from build123d import *

# Parameters (mm, degrees)
F0_R     = 19.05
F1_DEPTH = 3.302
F2_R     = 8.5345501525
F3_DEPTH = 6.605
F4_R     = 14.0253085835
F4_R_2   = 8.5345501525
F5_DEPTH = 0.762


# Not quite as in the source:
# - a feature names something its author has since deleted; it is built from what else it names


with BuildPart() as f1:
    # F0 (on Front) → F1 (new body, symmetric)
    with BuildSketch(Plane.XZ):
        Circle(F0_R)
    extrude(amount=F1_DEPTH, both=True)

    # F2 (on face) → F3 (cut, through all)
    with BuildSketch(Plane.XZ.offset(3.302)):
        Circle(F2_R)
    extrude(amount=-F3_DEPTH, mode=Mode.SUBTRACT)

    # F4 (on face) → F5 (cut)
    with BuildSketch(Plane.XZ.offset(3.302)):
        Circle(F4_R)
        Circle(F4_R_2, mode=Mode.SUBTRACT)
    extrude(amount=-F5_DEPTH, mode=Mode.SUBTRACT)


solid = f1.part
Verification items for the finished model (mm, model axes). A direction names the side the tool comes from. Coordinates: 2 decimals unless noted, no trailing zeros. Loops run counter-clockwise (first coordinate to the right, second up) from the corner with the lowest first, then second, coordinate; pieces in that order, holes last. Notation, with made-up numbers: (88, 69.25) -> (95, 69.25) arc R22 ccw to (95, 86.25) -> close; hole circle Ø2 at (42, 28.25). An arc over 180 degrees is marked (long way). Answer as a JSON object with one key per item and string values. Group by question number.
Item 1: Scan lines: probe 1 along Z at (x, y) = (0, 0.5); probe 2 along Z at (x, y) = (0, -2.9); probe 3 along Y at (x, z) = (-6.5, 9). Record each from-to range of solid material in increasing order.
Item 2: Sectioned sample at C-C on y = 1.5. Record the boundary of the cut face in (x, z).
Item 3: Tool access check on faces 4 (the cylindrical face through (12.956, -2.926, -5.372)), 5 (the flat face through (-9, -3.302, -11)). Record the directions out of +Z, -Z, +X, -X, +Y, -Y that give a thin tool (end or side, any length) a straight path to the whole face; none if there is none.
Item 4: Mould release check, pull along Z, two halves, no side actions. Record for faces 1 (the cylindrical face through (-15.12, -0.05, -11.59)), 2 (the flat face through (8, 3.302, -4)), 3 (the flat face through (0, -2.54, -9)): +Z half, -Z half, draft (parallel to the pull), parting line (faces both ways), or undercut.
Item 5: Sectioned sample at B-B on z = 0. Record the boundary of the cut face in (x, y).
Item 6: Depth check by flat-ended pin: pin 1 (8 mm diameter, centred on x = 8, z = 9, fed in from -Y); pin 2 (1.5 mm diameter, centred on x = 1.5, z = 10.5, fed in from -Y); pin 3 (3 mm diameter, centred on y = -1.5, z = -13, fed in from -X). Enter the tip coordinate at first touch or a pass-through.
Item 7: Sectioned sample at D-D on x = 10. Record the boundary of the cut face in (y, z), plus the area to 3 significant figures.
Item 8: Sectioned sample at A-A on x = 0. Record the boundary of the cut face in (y, z), plus the area to 3 significant figures.
Evaluation:
{
 "1": {"probe 1": "z = -19.05 to -8.53, 8.53 to 19.05", "probe 2": "z = -19.05 to -14.03, 14.03 to 19.05", "probe 3": "y = -2.54 to 3.3"},
 "2": {"outline": "circle Ø38.1 at (0, 0); hole circle Ø17.07 at (0, 0)"},
 "3": {"face 4": "-Y", "face 5": "+Z, -Z, +X, -X, -Y"},
 "4": {"face 1": "parting line", "face 2": "draft", "face 3": "undercut"},
 "5": {"outline": "(-19.05, -3.3) -> (-14.03, -3.3) -> (-14.03, -2.54) -> (-8.53, -2.54) -> (-8.53, 3.3) -> (-19.05, 3.3) -> close; (8.53, -2.54) -> (14.03, -2.54) -> (14.03, -3.3) -> (19.05, -3.3) -> (19.05, 3.3) -> (8.53, 3.3) -> close"},
 "6": {"pin 1": "stops at y = -3.3", "pin 2": "stops at y = -2.54", "pin 3": "stops at x = -15.19"},
 "7": {"outline": "(-3.3, -16.21) -> (3.3, -16.21) -> (3.3, 16.21) -> (-3.3, 16.21) -> (-3.3, 9.83) -> (-2.54, 9.83) -> (-2.54, -9.83) -> (-3.3, -9.83) -> close", "area": "199 mm²"},
 "8": {"outline": "(-3.3, -19.05) -> (3.3, -19.05) -> (3.3, -8.53) -> (-2.54, -8.53) -> (-2.54, -14.03) -> (-3.3, -14.03) -> close; (-3.3, 14.03) -> (-2.54, 14.03) -> (-2.54, 8.53) -> (3.3, 8.53) -> (3.3, 19.05) -> (-3.3, 19.05) -> close", "area": "131 mm²"}
}
